Could you check a few things on this model? Use its own coordinates, in mm. A direction names the side the tool comes from. Give positions to 0.01 mm unless a question says otherwise; leave off trailing zeros. Order: outer loops, then holes, each group sorted by start corner. A loop starts at its lowest first (then second) coordinate and runs counter-clockwise, first axis right, second up. Notation, with made-up numbers: M 66,24.5 L 79,24.5 A25 ccw 79,36.5 Z; hole C -6,62.25 d9. An arc over 180 degrees is marked long. Return JSON: item names as keys, results as strings. Group by question number.
```python
from build123d import *

# Parameters (mm, degrees)
SKETCH1_R           = 1.6
BOSS_EXTRUDE1_DEPTH = 3
SKETCH3_R           = 1.6
CUT_EXTRUDE2_DEPTH  = 4
CUT_EXTRUDE5_DEPTH  = 4
FILLET1_R           = 3.54


with BuildPart() as part:
    # Sketch1 → Boss-Extrude1 (new body)
    with BuildSketch(Plane.XY):
        with BuildLine():
            Line((-107, 98.923010333), (-107, -98.923010333))
            ThreePointArc((-107, -98.923010333), (-107.201661971, -101.11372249), (-107.799869959, -103.230804092))
            ThreePointArc((-107.799869959, -103.230804092), (-107, -107), (-103.230804092, -107.799869959))
            ThreePointArc((-103.230804092, -107.799869959), (-101.11372249, -107.201661971), (-98.923010333, -107))
            Line((-98.923010333, -107), (-43, -107))
            Line((-43, -107), (43, -107))
            Line((43, -107), (98.923010333, -107))
            ThreePointArc((98.923010333, -107), (101.11372249, -107.201661971), (103.230804092, -107.799869959))
            ThreePointArc((103.230804092, -107.799869959), (107, -107), (107.799869959, -103.230804092))
            ThreePointArc((107.799869959, -103.230804092), (107.201661971, -101.11372249), (107, -98.923010333))
            Line((107, -98.923010333), (107, 98.923010333))
            ThreePointArc((107, 98.923010333), (107.201661971, 101.11372249), (107.799869959, 103.230804092))
            ThreePointArc((107.799869959, 103.230804092), (107, 107), (103.230804092, 107.799869959))
            ThreePointArc((103.230804092, 107.799869959), (101.11372249, 107.201661971), (98.923010333, 107))
            Line((98.923010333, 107), (-98.923010333, 107))
            ThreePointArc((-98.923010333, 107), (-101.11372249, 107.201661971), (-103.230804092, 107.799869959))
            ThreePointArc((-103.230804092, 107.799869959), (-107, 107), (-107.799869959, 103.230804092))
            ThreePointArc((-107.799869959, 103.230804092), (-107.201661971, 101.11372249), (-107, 98.923010333))
        make_face()
        with Locations((-104.5, -104.5)):
            Circle(SKETCH1_R, mode=Mode.SUBTRACT)
        with Locations((-104.5, 104.5)):
            Circle(SKETCH1_R, mode=Mode.SUBTRACT)
        with Locations((104.5, 104.5)):
            Circle(SKETCH1_R, mode=Mode.SUBTRACT)
        with Locations((104.5, -104.5)):
            Circle(SKETCH1_R, mode=Mode.SUBTRACT)
    extrude(amount=BOSS_EXTRUDE1_DEPTH)

    # Sketch3 → Cut-Extrude2 (cut, through all)
    with BuildSketch(Plane.XY.offset(3)):
        with Locations((-71, 65)):
            Circle(SKETCH3_R)
        with Locations((71, 65)):
            Circle(SKETCH3_R)
        with Locations((71, -65)):
            Circle(SKETCH3_R)
        with Locations((-71, -65)):
            Circle(SKETCH3_R)
    extrude(amount=-CUT_EXTRUDE2_DEPTH, mode=Mode.SUBTRACT)

    # Sketch5 → Cut-Extrude5 (cut, through all)
    with BuildSketch(Plane.XY):
        with BuildLine():
            Line((-25, -107), (25, -107))
            Line((25, -107), (25, -69.5))
            ThreePointArc((25, -69.5), (23.535533906, -65.964466094), (20, -64.5))
            Line((20, -64.5), (14, -64.5))
            ThreePointArc((14, -64.5), (6.928932188, -61.571067812), (4, -54.5))
            Line((4, -54.5), (4, 0))
            ThreePointArc((4, 0), (0, 4), (-4, 0))
            Line((-4, 0), (-4, -54.5))
            ThreePointArc((-4, -54.5), (-6.928932188, -61.571067812), (-14, -64.5))
            Line((-14, -64.5), (-20, -64.5))
            ThreePointArc((-20, -64.5), (-23.535533906, -65.964466094), (-25, -69.5))
            Line((-25, -69.5), (-25, -107))
        make_face()
    extrude(amount=CUT_EXTRUDE5_DEPTH, mode=Mode.SUBTRACT)

    # Fillet1
    fillet1_edges = [part.edges().sort_by_distance(p)[0] for p in [
        (-25, -107, 1.5),
        (25, -107, 1.5),
    ]]
    fillet(fillet1_edges, radius=FILLET1_R)


solid = part.part
```
1. If we mould it in two halves opening along X, with no side actions, what happens to faces 3 (the flat face through (-2, 26, 3)), 4 (the cylindrical face through (-23.5, -65.93, 1.48))? For each: pulls with the +X half, pulls with the -X half, needs draft (parallel to the pull), parting line crosses it, or undercut.
2. Imagine slicing it at A-A, the plane y = -72.5. Please give me the cut outline in (x, z).
3. Imagine slicing it at C-C, the plane x = 0. Please give me the cut outline in (y, z).
4. Imagine slicing it at B-B, the plane z = 2.1. Count the separate pieces of the cut face and the enclosed holes in it, plus the area to 3 significant figures.
5. I need wall thicknesses on L1, parallel to X at y = 65, z = 1.1; L2, parallel to Y at x = 71, z = 0.65; L3, parallel to Y at x = -104.5, z = 2.05. Which ranges of each line are inside material? Lowest first, please. Write a range as from..to.
6. For pin 1 (1.5 mm diameter, centred on y = -17.5, z = 1, fed in from +X); pin 2 (1.5 mm diameter, centred on y = -82, z = 2, fed in from -X), each with a flat end and sliding along its axis, tell me the tip position at first contact or that it passes through.
7. Which directions (+Z, -Z, +X, -X, +Y, -Y) give clear straight access to the entire face, cutting with the end or side of a thin tool? Please do faces 1 (the flat face through (-2, 26, 0)), 2 (the cylindrical face through (7.01, -61.65, 1.48)).
Values:
{
 "1": {"face 3": "needs draft", "face 4": "undercut"},
 "2": {"outline": "M -107,0 L -25,0 L -25,3 L -107,3 Z; M 25,0 L 107,0 L 107,3 L 25,3 Z"},
 "3": {"outline": "M 4,0 L 107,0 L 107,3 L 4,3 Z"},
 "4": {"separate pieces": "1", "enclosed holes": "8", "area": "43,100 mm²"},
 "5": {"L1": "x = -107..-72.6, -69.4..69.4, 72.6..107", "L2": "y = -107..-66.6, -63.4..63.4, 66.6..107", "L3": "y = -108.04..-106.1, -102.9..102.9, 106.1..108.04"},
 "6": {"pin 1": "stops at x = 107", "pin 2": "stops at x = -107"},
 "7": {"face 1": "-Z, +X, -X, +Y, -Y", "face 2": "+Z, -Z, -Y"}
}
